```python
from build123d import *

# Parameters (mm, degrees)
F1_DEPTH = 2
F2_W     = 2
F2_H     = 14.964955
F3_DEPTH = 25


with BuildPart() as f1:
    # F0 (on Front) → F1 (new body)
    with BuildSketch(Plane.XZ):
        with BuildLine():
            ThreePointArc((0, 30), (-21.213203, 21.213203), (-30, 0))
            Line((-30, 0), (0, 0))
            Line((0, 0), (0, 30))
        make_face()
    extrude(amount=F1_DEPTH)

    # F2 (on Front) → F3 (cut)
    with BuildSketch(Plane.XZ):
        with Locations((-6, 22.482478)):
            Rectangle(F2_W, F2_H)
    extrude(amount=F3_DEPTH, mode=Mode.SUBTRACT)


solid = f1.part
```
For this review, take the finished solid that the model builds, in its own axes (mm). A direction names the side the tool comes from. Round coordinates to 2 decimals unless told otherwise and drop trailing zeros. Order: outer loops, then holes, each group sorted by start corner. A loop starts at its lowest first (then second) coordinate and runs counter-clockwise, first axis right, second up.
Q1. We need section A-A, the plane z = 21. Give the boundary of the cut face in (x, y), plus the area to 3 significant figures.
Findings below:
outline: (-21.42, -2) - (-7, -2) - (-7, 0) - (-21.42, 0) - close; (-5, -2) - (0, -2) - (0, 0) - (-5, 0) - close
area: 38.8 mm2
Q2. Wall thickness on line 1 (Z direction, x = -6, y = -1.1); line 2 (X direction, y = -1.25, z = 2.75); line 3 (X direction, y = -1.5, z = 10): over which ranges is each line inside the solid? List them lowest first.
Findings below:
line 1: z = 0 to 15
line 2: x = -29.87 to 0
line 3: x = -28.28 to 0
Q3. We need section D-D, the plane z = 26.75. Give the boundary of the cut face in (x, y), plus the area to 3 significant figures.
Findings below:
outline: (-13.58, -2) - (-7, -2) - (-7, 0) - (-13.58, 0) - close; (-5, -2) - (0, -2) - (0, 0) - (-5, 0) - close
area: 23.2 mm2
Q4. We need section B-B, the plane y = -0.85. Give the boundary of the cut face in (x, z).
Findings below:
outline: (-30, 0) - (0, 0) - (0, 30) arc R30 ccw to (-5, 29.58) - (-5, 15) - (-7, 15) - (-7, 29.17) arc R30 ccw to start
Q5. Insertion check: P1, Ø0.6, axis at x = -6.5, y = -0.5, coming from the +Z side; P2, Ø0.6, axis at y = -1, z = 24, coming from the -X side. Each pin has a flat end and moves straight along its axis. Give the tip position at first contact, or say it passes through.
Findings below:
P1: stops at z = 15
P2: stops at x = -18.39
Q6. Mouldability with a two-part tool opening along X and no side actions: class faces 1 (the flat face through (-15, -1, 0)), 2 (the flat face through (-7, -1, 22)), 3 (the cylindrical face through (-23.384, -0.986, 18.794)) as pulls with the +X half, pulls with the -X half, needs draft (parallel to the pull), parting line crosses it, or undercut.
Findings below:
face 1: needs draft
face 2: undercut
face 3: pulls with the -X half
Q7. Machinability: for faces 4 (the flat face through (-6, -1, 15)), 5 (the flat face through (0, -1, 15)), which of the approach directions +Z, -Z, +X, -X, +Y, -Y give a long, thin tool a straight path to every point of the face, cutting with its end or side? Answer none if there is none.
Findings below:
face 4: +Z, +Y, -Y
face 5: +Z, -Z, +X, +Y, -Y
Q8. We need section C-C, the plane x = -18. Give the boundary of the cut face in (y, z), plus the area to 3 significant figures.
Findings below:
outline: (-2, 0) - (0, 0) - (0, 24) - (-2, 24) - close
area: 48.0 mm2
